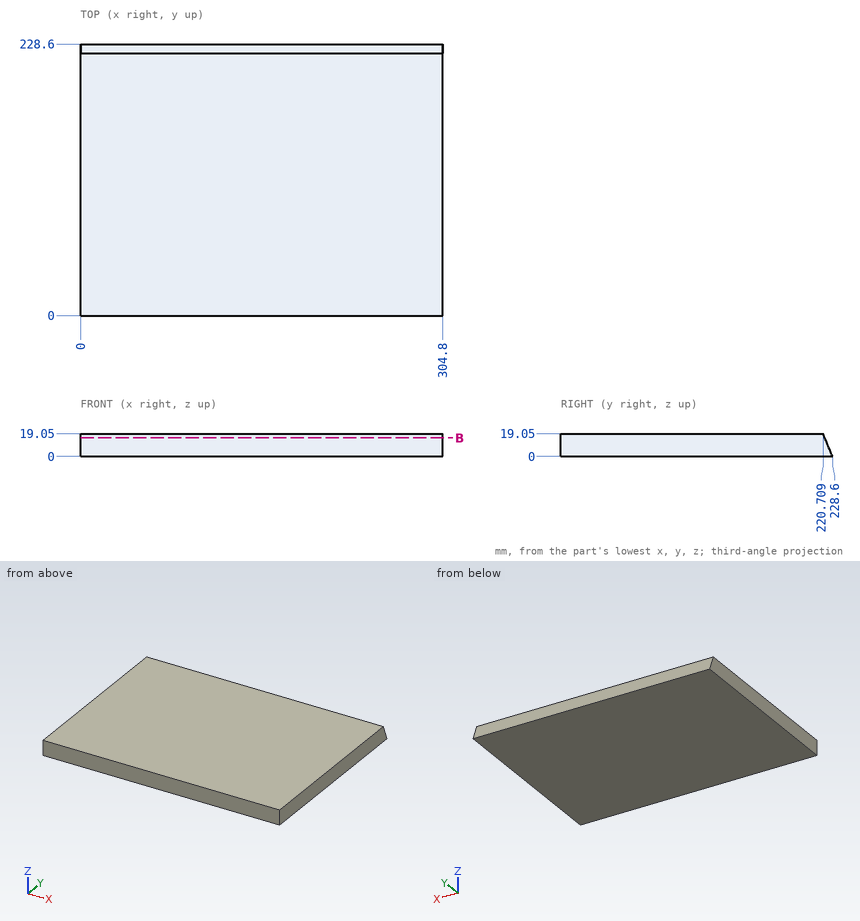
Input: dimensioned drawing with shaded views. Units: mm. Origin: part minimum x, y, z. Round coordinates to 2 decimals unless told otherwise and drop trailing zeros. Loops run counter-clockwise (first coordinate to the right, second up) from the corner with the lowest first, then second, coordinate; pieces in that order, holes last. Notation, with made-up numbers: (-25.75, 71.25) -> (5.25, 71.25) arc R23 cw to (5.25, 92.25) -> close; hole circle Ø5 at (19, -27.5). An arc over 180 degrees is marked (long way). Use one line per item in the form item = value. Start each with the question number.
1) Line query: L1, parallel to Y at x = 250, z = 8; L2, parallel to Y at x = 167.5, z = 17. Output: solid intervals per line, ascending.
2) First-contact query: P1, Ø3, axis at x = 258, z = 7, coming from the +Y side. Flat tip, straight axial feed; report the tip coordinate or a pass-through.
3) Section B-B on z = 15.5. Output: boundary loops of the cut face in (x, y), then the cut area to 3 significant figures.
Response:
q1.L1 = 0 to 225.29
q1.L2 = 0 to 221.56
q2.P1 = 226.32
q3.outline = (0, 0) -> (304.8, 0) -> (304.8, 222.18) -> (0, 222.18) -> close
q3.area = 67,700 mm^2
